```python
from build123d import *

# Parameters (mm, degrees)
ESQUISSE1_W             = 27.85
ESQUISSE1_H             = 40
BOSS_EXTRU_1_DEPTH      = 6
ESQUISSE2_R             = 13.925
ENL_V_MAT_EXTRU_1_DEPTH = 3


with BuildPart() as part:
    # Esquisse1 → Boss.-Extru.1 (new body)
    with BuildSketch(Plane(origin=(0, 0, 0), x_dir=(0, 0, -1), z_dir=(1, 0, 0))):
        with Locations((-1.440517241, 18.893965517)):
            Rectangle(ESQUISSE1_W, ESQUISSE1_H)
        with BuildLine():
            ThreePointArc((12.484482759, -1.106034483), (-1.440517241, -15.031034483), (-15.365517241, -1.106034483))
            Line((-15.365517241, -1.106034483), (12.484482759, -1.106034483))
        make_face()
    extrude(amount=BOSS_EXTRU_1_DEPTH)

    # Esquisse2 → Enlèv. mat.-Extru.1 (cut)
    with BuildSketch(Plane(origin=(6, 0, 0), x_dir=(0, 0, -1), z_dir=(1, 0, 0))):
        with Locations((-1.440517241, -1.106034483)):
            Circle(ESQUISSE2_R)
    extrude(amount=-ENL_V_MAT_EXTRU_1_DEPTH, mode=Mode.SUBTRACT)


solid = part.part
```
Model file for the job. Use its own axes, mm. A direction names the side the tool comes from. Coordinates: 2 decimals unless noted, no trailing zeros. Order: outer loops, then holes, each group sorted by start corner. A loop starts at its lowest first (then second) coordinate and runs counter-clockwise, first axis right, second up. Notation, with made-up numbers: M 89,0.25 L 134,0.25 A32 cw 134,34.25 Z; hole C 83.25,-37 d4. An arc over 180 degrees is marked long. Answer as CSV lines item,"result".
(1) Band-saw the part on C-C, the plane z = 10.5. List the corners of the cut face in (x, y), then the cut area to 3 significant figures.
Geometry says:
outline,"M 0,-11.68 L 3,-11.68 L 3,9.47 L 6,9.47 L 6,38.89 L 0,38.89 Z"
area,"240 mm2"
(2) Wall check: line 1 along X through (y, z) = (8, 5); line 2 along Y through (x, z) = (2.2, 3); line 3 along Z through (x, y) = (4.6, 11). Give the ranges that are in metal, low to high.
Geometry says:
line 1,"x = 0 to 3"
line 2,"y = -14.94 to 38.89"
line 3,"z = -12.48 to -5.44, 8.32 to 15.37"
(3) 3-axis set-ups, long thin cutter, end or side, ignore diameter. For faces 1 (the flat face through (3, -1, 2)), 2 (the flat face through (0, 12, 2)): which of +Z, -Z, +X, -X, +Y, -Y reach the whole face in a straight line?
Geometry says:
face 1,"+X, -Y"
face 2,"+Z, -Z, -X, +Y, -Y"
(4) Band-saw the part on D-D, the plane x = 0.55. List the corners of the cut face in (y, z) (3 decimals), then the cut area to 3 significant figures.
Geometry says:
outline,"M -1.106,-12.484 L 38.894,-12.484 L 38.894,15.366 L -1.106,15.366 A13.925 ccw Z"
area,"1,420 mm2"
(5) Band-saw the part on A-A, the plane y = 5. List the corners of the cut face in (x, z), then the cut area to 3 significant figures.
Geometry says:
outline,"M 0,-12.48 L 6,-12.48 L 6,-11.07 L 3,-11.07 L 3,13.96 L 6,13.96 L 6,15.37 L 0,15.37 Z"
area,"92.0 mm2"
(6) Flat gauge pin, fed straight in: pin 1 (6 mm diameter, centred on y = -4, z = -9.5, fed in from +X). Where does the tip first touch, or does it go through?
Geometry says:
pin 1,"stops at x = 3"
(7) Band-saw the part on B-B, the plane x = 3.85. List the corners of the cut face in (y, z) (3 decimals), then the cut area to 3 significant figures.
Geometry says:
outline,"M -1.106,-12.484 L 38.894,-12.484 L 38.894,15.366 L -1.106,15.366 A13.925 cw Z"
area,"809 mm2"
